Can you work these out from the model? Positions are in its coordinate system, mm. Face numbers are marked on the shaded views. Round coordinates to 2 decimals unless told otherwise and drop trailing zeros. Order: outer loops, then holes, each group sorted by start corner. A loop starts at its lowest first (then second) coordinate and runs counter-clockwise, first axis right, second up. Notation, with made-up numbers: M 54,45 L 67,45 A19 ccw 67,82 Z; hole C -22,-23 d10. An arc over 180 degrees is marked long. Answer as a JSON object with one key per item and string values. Group by question number.
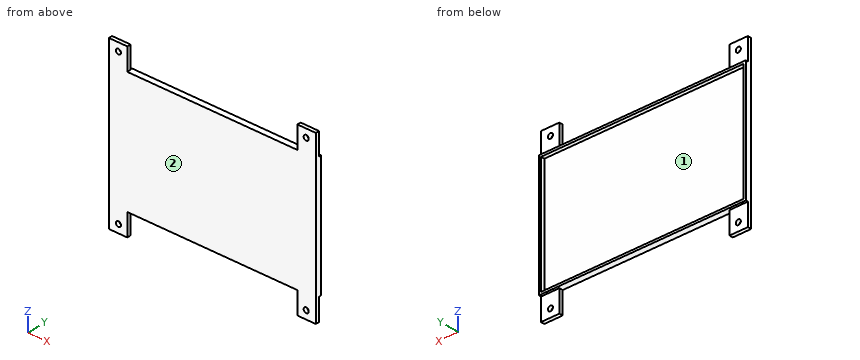
from build123d import *

# Parameters (mm, degrees)
SKETCH1_W           = 280
SKETCH1_H           = 165.1
BOSS_EXTRUDE1_DEPTH = 3.175
SKETCH2_W           = 280
SKETCH2_H           = 165.1
SKETCH2_W_2         = 274
SKETCH2_H_2         = 159.1
BOSS_EXTRUDE2_DEPTH = 5
SKETCH3_W           = 25
SKETCH3_H           = 30
SKETCH3_R           = 3.429
BOSS_EXTRUDE3_DEPTH = 5


with BuildPart() as part:
    # Sketch1 → Boss-Extrude1 (new body)
    with BuildSketch(Plane(origin=(0, 0, 0), x_dir=(1, 0, 0), z_dir=(0, 1, 0))):
        Rectangle(SKETCH1_W, SKETCH1_H)
    extrude(amount=BOSS_EXTRUDE1_DEPTH)

    # Sketch2 → Boss-Extrude2 (add)
    with BuildSketch(Plane(origin=(0, 3.175, 0), x_dir=(1, 0, 0), z_dir=(0, 1, 0))):
        Rectangle(SKETCH2_W, SKETCH2_H)
        Rectangle(SKETCH2_W_2, SKETCH2_H_2, mode=Mode.SUBTRACT)
    extrude(amount=BOSS_EXTRUDE2_DEPTH)

    # Sketch3 → Boss-Extrude3 (add)
    # profile 1 of 4: a face of its own
    with BuildSketch(Plane(origin=(0, 0, 0), x_dir=(1, 0, 0), z_dir=(0, 1, 0))):
        with Locations((-127.5, 97.55)):
            Rectangle(SKETCH3_W, SKETCH3_H)
        with Locations(Location((-127, 101.6, 0), (0, 0, 270))):
            Circle(SKETCH3_R, mode=Mode.SUBTRACT)
    # profile 2 of 4: a face of its own
    with BuildSketch(Plane(origin=(0, 0, 0), x_dir=(1, 0, 0), z_dir=(0, 1, 0))):
        with Locations((127.5, 97.55)):
            Rectangle(SKETCH3_W, SKETCH3_H)
        with Locations(Location((127, 101.6, 0), (0, 0, 270))):
            Circle(SKETCH3_R, mode=Mode.SUBTRACT)
    # profile 3 of 4: a face of its own
    with BuildSketch(Plane(origin=(0, 0, 0), x_dir=(1, 0, 0), z_dir=(0, 1, 0))):
        with Locations((-127.5, -97.55)):
            Rectangle(SKETCH3_W, SKETCH3_H)
        with Locations(Location((-127, -101.6, 0), (0, 0, 270))):
            Circle(SKETCH3_R, mode=Mode.SUBTRACT)
    # profile 4 of 4: a face of its own
    with BuildSketch(Plane(origin=(0, 0, 0), x_dir=(1, 0, 0), z_dir=(0, 1, 0))):
        with Locations((127.5, -97.55)):
            Rectangle(SKETCH3_W, SKETCH3_H)
        with Locations(Location((127, -101.6, 0), (0, 0, 270))):
            Circle(SKETCH3_R, mode=Mode.SUBTRACT)
    extrude(amount=BOSS_EXTRUDE3_DEPTH)


solid = part.part
Item 1: Suppose I cut it at D-D, the plane y = 1.5. Write out the boundary of the cut face in (x, z).
Item 2: Suppose I cut it at B-B, the plane z = -101.6. Write out the boundary of the cut face in (x, y).
Item 3: I need wall thicknesses on line 1 (X direction, y = 3.95, z = -101.6); line 2 (Z direction, x = 89, y = 7); line 3 (X direction, y = 5, z = -31). Which ranges of each line are inside material? Lowest first, please.
Item 4: I'm going to push flat-ended pins straight in: pin 1 Ø1.5 at (x, y) = (-38.5, 5.5) entering from -Z; pin 2 Ø4 at (x, z) = (-69.5, -51) entering from +Y (3 decimals); pin 3 Ø20 at (x, z) = (-122.5, 99.5) entering from +Y. Where does each tip first touch, or does it pass through?
Item 5: If we mould it in two halves opening along Z, with no side actions, what happens to the marked faces 1 and 2? For each: +Z half, -Z half, draft (parallel to the pull), parting line (faces both ways), or undercut.
Item 6: Suppose I cut it at A-A, the plane x = 127. Write out the boundary of the cut face in (y, z) (3 decimals), and give its area (3 significant figures).
Item 7: Suppose I cut it at C-C, the plane x = -23. Write out the boundary of the cut face in (y, z) (3 decimals), and give its area (3 significant figures).
Computed:
{
 "1": {"outline": "M -140,-112.55 L -115,-112.55 L -115,-82.55 L 115,-82.55 L 115,-112.55 L 140,-112.55 L 140,112.55 L 115,112.55 L 115,82.55 L -115,82.55 L -115,112.55 L -140,112.55 Z; hole C -127,-101.6 d6.86; hole C -127,101.6 d6.86; hole C 127,-101.6 d6.86; hole C 127,101.6 d6.86"},
 "2": {"outline": "M -140,0 L -130.43,0 L -130.43,5 L -140,5 Z; M -123.57,0 L -115,0 L -115,5 L -123.57,5 Z; M 115,0 L 123.57,0 L 123.57,5 L 115,5 Z; M 130.43,0 L 140,0 L 140,5 L 130.43,5 Z"},
 "3": {"line 1": "x = -140 to -130.43, -123.57 to -115, 115 to 123.57, 130.43 to 140", "line 2": "z = -82.55 to -79.55, 79.55 to 82.55", "line 3": "x = -140 to -137, 137 to 140"},
 "4": {"pin 1": "stops at z = -82.55", "pin 2": "stops at y = 3.175", "pin 3": "stops at y = 5"},
 "5": {"face 1": "undercut", "face 2": "draft"},
 "6": {"outline": "M 0,-112.55 L 5,-112.55 L 5,-105.029 L 0,-105.029 Z; M 0,-98.171 L 5,-98.171 L 5,-82.55 L 8.175,-82.55 L 8.175,-79.55 L 3.175,-79.55 L 3.175,79.55 L 8.175,79.55 L 8.175,82.55 L 5,82.55 L 5,98.171 L 0,98.171 Z; M 0,105.029 L 5,105.029 L 5,112.55 L 0,112.55 Z", "area": "786 mm^2"},
 "7": {"outline": "M 0,-82.55 L 8.175,-82.55 L 8.175,-79.55 L 3.175,-79.55 L 3.175,79.55 L 8.175,79.55 L 8.175,82.55 L 0,82.55 Z", "area": "554 mm^2"}
}
